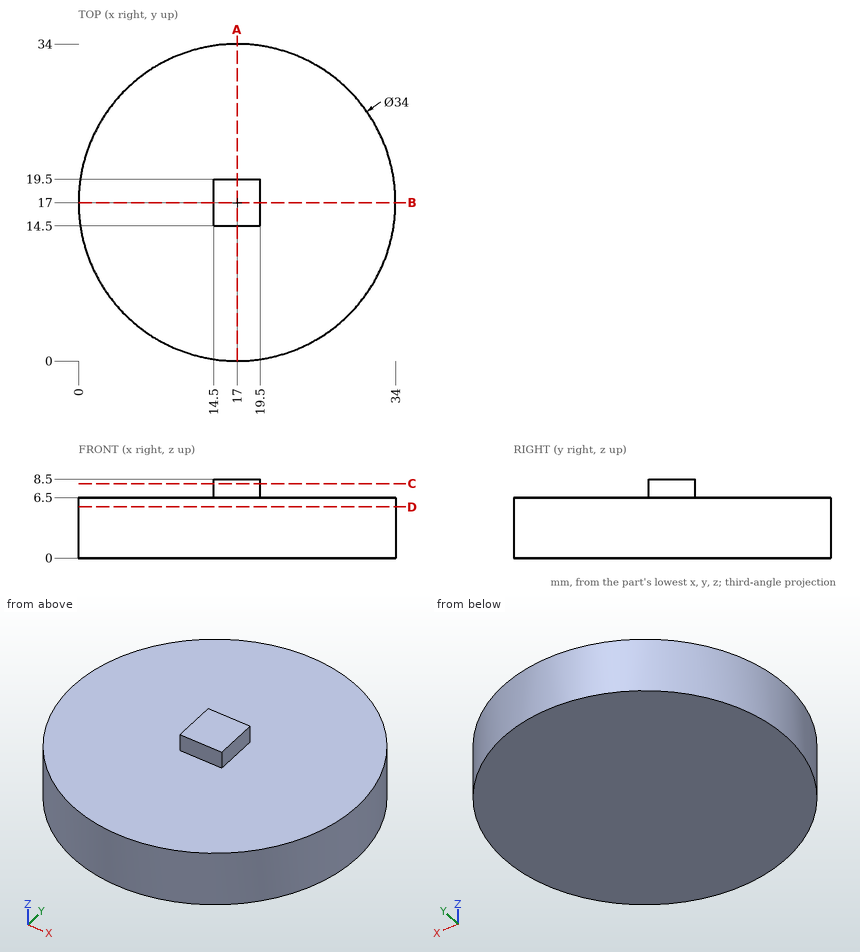
Study the drawing (mm; zero at the part's minimum x, y, z) and answer. Coordinates: 2 decimals unless noted, no trailing zeros. Write each loop counter-clockwise with the first axis right and the second up, starting at its lowest first coordinate (ties: lowest second). Pieces come first, ordered by that corner, then holes.
Q1. A cutting plane is placed at C-C, the plane z = 8. Give the vertices of the cut face in (x, y), then the cut area to 3 significant figures.
Q2. A cutting plane is placed at D-D, the plane z = 5.5. Give the vertices of the cut face in (x, y), then the cut area to 3 significant figures.
Q3. Find the intervals of material crossed by line 1 (Z direction, x = 31.5, y = 8.5); line 2 (Y direction, x = 16, z = 7), in increasing order.
Q4. Each of these flat-tipped pins is pushed along its axis until it touches: pin 1 Ø1.5 at (x, z) = (18.5, 7) entering from +Y; pin 2 Ø1.6 at (x, z) = (16, 7.5) entering from -Y; pin 3 Ø0.6 at (x, z) = (16.5, 7.5) entering from +Y; pin 4 Ø17 at (x, y) = (13, 23) entering from +Z. Where does it stop, or does it pass through?
Q5. A cutting plane is placed at A-A, the plane x = 17. Give the vertices of the cut face in (y, z), then the cut area to 3 significant figures.
Findings below:
1. outline: (14.5, 14.5) - (19.5, 14.5) - (19.5, 19.5) - (14.5, 19.5) - close
1. area: 25.0 mm2
2. outline: circle Ø34 at (17, 17)
2. area: 908 mm2
3. line 1: z = 0 to 6.5
3. line 2: y = 14.5 to 19.5
4. pin 1: stops at y = 33.97
4. pin 2: stops at y = 14.5
4. pin 3: stops at y = 19.5
4. pin 4: stops at z = 8.5
5. outline: (0, 0) - (34, 0) - (34, 6.5) - (19.5, 6.5) - (19.5, 8.5) - (14.5, 8.5) - (14.5, 6.5) - (0, 6.5) - close
5. area: 231 mm2
